```python
from build123d import *

# Parameters (mm, degrees)
F1_DEPTH      = 254
F1_DEPTH_BACK = 254
F3_D          = 6.35
F4_R          = 49.5981028819
F4_R_2        = 3.175
F5_DEPTH      = 25.4
F6_DEPTH      = 25.4
F7_DEPTH      = 25.4


with BuildPart() as f1:
    # F0 (on Top) → F1 (new body, two sides)
    with BuildSketch(Plane.XY) as f1_sk:
        Polygon((-51.0406941175, 0), (0, 0), (0, -58.7314069271), (56.7247420549, -58.7314069271), (56.7247420549, -17.6112949848), (87.1720016003, -17.6112949848), (87.1720016003, 139.7417336702), (29.5281931758, 139.7417336702), (29.5281931758, 98.9419966936), (-51.0406941175, 98.9419966936), align=None)
    extrude(amount=F1_DEPTH)
    extrude(f1_sk.sketch, amount=-F1_DEPTH_BACK)

    # F3 (through all)
    with Locations(Plane.YZ.offset(87.1720016003)):
        with Locations((71.7472732067, 138.4787261486), (50.1599907875, 0)):
            Hole(F3_D / 2)

    # F4 (on face) → F5 (cut)
    with BuildSketch(Plane.YZ.offset(87.1720016003)):
        with Locations((71.7472732067, 138.4787261486)):
            Circle(F4_R)
        with Locations((71.7472732067, 138.4787261486)):
            Circle(F4_R_2, mode=Mode.SUBTRACT)
    extrude(amount=-F5_DEPTH, mode=Mode.SUBTRACT)

    # F6 (cut): a face of the model
    f6_faces = [f1.faces().sort_by_distance(p)[0] for p in [
        (26.0044573743, 42.9582236977, 254),
    ]]
    extrude(f6_faces, amount=-F6_DEPTH, mode=Mode.SUBTRACT)

    # F7 (cut): a face of the model
    f7_faces = [f1.faces().sort_by_distance(p)[0] for p in [
        (87.1720016003, 59.8594463551, -29.8423997795),
    ]]
    extrude(f7_faces, amount=-F7_DEPTH, mode=Mode.SUBTRACT)


solid = f1.part
```
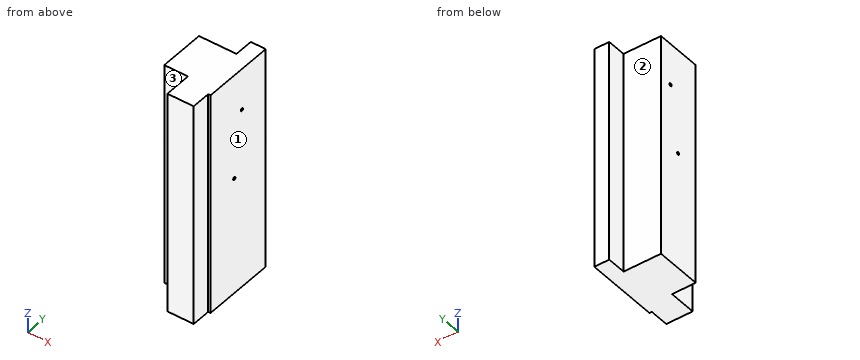
Model file for the job. Use its own axes, mm. Face numbers are marked on the shaded views. A direction names the side the tool comes from. Coordinates: 2 decimals unless noted, no trailing zeros. Loops run counter-clockwise (first coordinate to the right, second up) from the corner with the lowest first, then second, coordinate; pieces in that order, holes last. Notation, with made-up numbers: (30, 17) - (52, 17) arc R26 ccw to (52, 43) - close; hole circle Ø2 at (-1, 16.5). An arc over 180 degrees is marked (long way). Answer as a JSON object with one key per item and string values. Group by question number.
(1) Cut at C-C (x = 16). Give the cut face in (y, z) (3 decimals), then the cut area to 3 significant figures.
(2) Tool access for the marked faces 1, 2 and 3: list every direction of +Z, -Z, +X, -X, +Y, -Y with a clear straight run to the whole face (end or side of a thin tool).
(3) Cut at D-D (x = -23). Give the cut face in (y, z) (3 decimals).
(4) Cut at B-B (y = -24). Give the cut face in (x, z).
(5) Cut at A-A (z = -88). Give the cut face in (x, y), then the cut area to 3 significant figures.
(6) Flat gauge pins, fed straight in: pin 1 (12 mm diameter, centred on y = -30, z = -91, fed in from -X); pin 2 (1.5 mm diameter, centred on x = 60, z = -51, fed in from -Y); pin 3 (12 mm diameter, centred on x = 4.5, z = 45.5, fed in from +Y). Where does each tip first touch, or does it go through?
(7) Probe line 1 along Y through (x, z) = (-25, -200); line 2 along X through (y, z) = (-4, -28.5); line 3 along X through (y, z) = (-45, -99). List the from-to ranges inside material, lowest first.
Geometry says:
{
 "1": {"outline": "(-58.731, -254) - (98.942, -254) - (98.942, 228.6) - (-58.731, 228.6) - close; hole circle Ø6.35 at (50.16, 0); hole circle Ø6.35 at (71.747, 138.479)", "area": "76,000 mm^2"},
 "2": {"face 1": "+Z, -Z, +X, +Y, -Y", "face 2": "+Z, -Z, -X, +Y", "face 3": "+Z, -Z, -X, -Y"},
 "3": {"outline": "(0, -254) - (98.942, -254) - (98.942, 228.6) - (0, 228.6) - close; hole circle Ø6.35 at (50.16, 0); hole circle Ø6.35 at (71.747, 138.479)"},
 "4": {"outline": "(0, -254) - (56.72, -254) - (56.72, 228.6) - (0, 228.6) - close"},
 "5": {"outline": "(-51.04, 0) - (0, 0) - (0, -58.73) - (56.72, -58.73) - (56.72, -17.61) - (61.77, -17.61) - (61.77, 139.74) - (29.53, 139.74) - (29.53, 98.94) - (-51.04, 98.94) - close", "area": "15,900 mm^2"},
 "6": {"pin 1": "stops at x = 0", "pin 2": "stops at y = -17.61", "pin 3": "stops at y = 98.94"},
 "7": {"line 1": "y = 0 to 98.94", "line 2": "x = 0 to 61.77", "line 3": "x = 0 to 56.72"}
}
